Geometry: final body of the model. Coordinates: model frame, mm. Face numbers are marked on the shaded views. A direction names the side the tool comes from. Round coordinates to 2 decimals unless told otherwise and drop trailing zeros. Order: outer loops, then holes, each group sorted by start corner. A loop starts at its lowest first (then second) coordinate and runs counter-clockwise, first axis right, second up. Notation, with made-up numbers: M 54,24.25 L 62,24.25 A29 cw 62,47.25 Z; hole C 3.25,39.25 d11. An arc over 180 degrees is marked long. Return JSON: item names as keys, results as strings. Group by question number.
Q1. Cut plane A-A on y = 38. Output: boundary loops of the cut face in (x, z), and give its area (3 significant figures).
Q2. Cut plane C-C on z = -2.5. Output: boundary loops of the cut face in (x, y), and give its area (3 significant figures).
Q3. Mould query, pull axis Z, two halves, no side actions, for the marked faces 6, 7, 8 and 9. Classes: released by +Z, released by -Z, zero draft, split by the parting line, or undercut.
Q4. Contact query for flat-ended pins moving along their axis: pin 1 (2 mm diameter, centred on x = 73, y = 13.5, fed in from +Z); pin 2 (12 mm diameter, centred on x = 97.5, z = 10.5, fed in from -Y); pin 3 (2 mm diameter, centred on x = 101.5, z = 2, fed in from +Y); pin 4 (12 mm diameter, centred on x = 16.5, z = 5, fed in from +Y). Output: stop coordinate, or through.
Q5. Ray query, probe 1 along Z at (x, y) = (6, 33); probe 2 along Y at (x, z) = (59, -6); probe 3 along Y at (x, z) = (36.5, 4.5). Return the intervals inside material, ascending.
Q6. Cut plane B-B on x = 59. Output: boundary loops of the cut face in (y, z).
Q7. Cut plane D-D on y = 13. Output: boundary loops of the cut face in (x, z), and give its area (3 significant figures).
Q8. Access query for the marked faces 1, 2, 3, 4 and 5. Directions: +Z, -Z, +X, -X, +Y, -Y. A direction counts if a zero-diameter tool reaches every point of the face in a straight line with its end or side. Return the directions, or none.
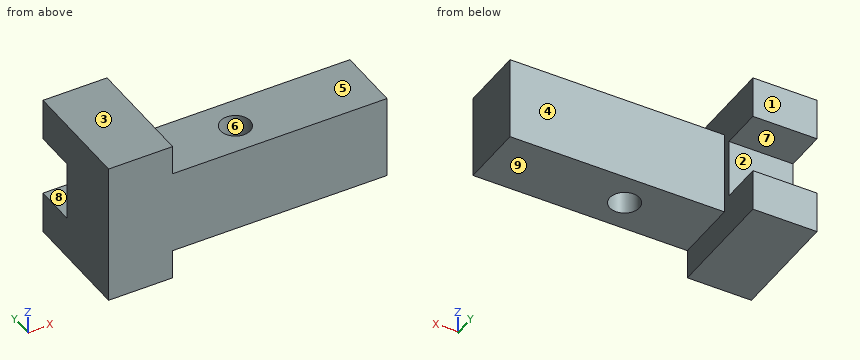
```python
from build123d import *

# Parameters (mm, degrees)
EXTRUDE_1_DEPTH = 26
SKETCH_2_W      = 87
SKETCH_2_H      = 26
SKETCH_2_R      = 6
EXTRUDE_2_DEPTH = 17


with BuildPart() as part:
    # 스케치1 → 보스-돌출1 (new body)
    with BuildSketch(Plane(origin=(0, 0, 0), x_dir=(0, 0, -1), z_dir=(1, 0, 0))):
        Polygon((-29, 0), (29, 0), (29, 46), (12, 46), (12, 29.19214502), (-12, 29.19214502), (-12, 46), (-29, 46), align=None)
    extrude(amount=EXTRUDE_1_DEPTH)

    # 스케치2 → 보스-돌출2 (add, symmetric)
    with BuildSketch(Plane.XY):
        with Locations((69.5, 13)):
            Rectangle(SKETCH_2_W, SKETCH_2_H)
        with Locations((59, 13)):
            Circle(SKETCH_2_R, mode=Mode.SUBTRACT)
    extrude(amount=EXTRUDE_2_DEPTH, both=True)


solid = part.part
```
Result sheet:
{
 "1": {"outline": "M 0,-29 L 26,-29 L 26,-12 L 0,-12 Z; M 0,12 L 26,12 L 26,29 L 0,29 Z", "area": "884 mm²"},
 "2": {"outline": "M 0,0 L 113,0 L 113,26 L 26,26 L 26,29.19 L 0,29.19 Z; hole C 59,13 d12", "area": "2,910 mm²"},
 "3": {"face 6": "zero draft", "face 7": "undercut", "face 8": "undercut", "face 9": "released by -Z"},
 "4": {"pin 1": "stops at z = 17", "pin 2": "stops at y = 0", "pin 3": "stops at y = 26", "pin 4": "stops at y = 29.19"},
 "5": {"probe 1": "z = -29 to -12, 12 to 29", "probe 2": "y = 0 to 7, 19 to 26", "probe 3": "y = 0 to 26"},
 "6": {"outline": "M 0,-17 L 7,-17 L 7,17 L 0,17 Z; M 19,-17 L 26,-17 L 26,17 L 19,17 Z"},
 "7": {"outline": "M 0,-29 L 26,-29 L 26,-17 L 53,-17 L 53,17 L 26,17 L 26,29 L 0,29 Z; M 65,-17 L 113,-17 L 113,17 L 65,17 Z", "area": "4,060 mm²"},
 "8": {"face 1": "+Z, -Z, +X, -X, +Y", "face 2": "+X, -X, +Y", "face 3": "+Z, +X, -X, +Y, -Y", "face 4": "+Z, -Z, +X, +Y", "face 5": "+Z, +X, +Y, -Y"}
}
